```python
from build123d import *

# Parameters (mm, degrees)
SKETCH1_W                                    = 25.4
SKETCH1_H                                    = 6.35
BOSS_EXTRUDE3_DEPTH                          = 6.35
BOSS_EXTRUDE5_DEPTH                          = 6.35
CBORE_FOR_M3_HEX_SOCKET_HEAD_CAP_SCR_2_COUNT = 2
CBORE_FOR_M3_HEX_SOCKET_HEAD_CAP_SCR_2_PITCH = 50.8
CIRPATTERN1_COUNT                            = 5
F_3_0MM_DOWEL_HOLE1_D                        = 3
F_3_0MM_DOWEL_HOLE1_CSINK_D                  = 3.05
F_3_0MM_DOWEL_HOLE1_CSINK_ANGLE              = 90


with BuildPart() as part:
    # Sketch1 → Boss-Extrude3 (new body)
    with BuildSketch(Plane.XY):
        Polygon((-124.216211638, 59.788282184), (-139.456211638, 80.108282184), (-159.776211638, 64.868282184), (-144.536211638, 44.548282184), (-168.571099043, 36.333406201), (-160.356223061, 12.298518796), (-136.321335655, 20.513394779), (-128.106459673, -3.521492627), (-152.141347078, -11.73636861), (-143.926471095, -35.771256015), (-119.89158369, -27.556380032), (-111.676707707, -51.591267438), (-135.711595113, -59.80614342), (-127.49671913, -83.841030826), (-103.461831725, -75.626154843), (-95.246955742, -99.661042248), (-119.281843147, -107.875918231), (-111.066967165, -131.910805636), (-87.032079759, -123.695929654), (-86.646457092, -149.093002224), (-61.249384521, -148.707379557), (-61.635007189, -123.310306986), (-36.237934618, -122.924684318), (-35.85231195, -148.321756889), (-10.45523938, -147.936134221), (-10.840862048, -122.539061651), (14.556210523, -122.153438983), (14.941833191, -147.550511554), (40.338905761, -147.164888886), (39.953283094, -121.767816315), (65.350355664, -121.382193648), (65.735978332, -146.779266218), (91.133050903, -146.393643551), (90.747428235, -120.99657098), (115.020643556, -128.477949061), (122.502021637, -104.20473374), (98.228806316, -96.723355659), (105.710184397, -72.450140338), (129.983399717, -79.931518419), (137.464777798, -55.658303098), (113.191562477, -48.176925017), (120.672940558, -23.903709697), (144.946155879, -31.385087777), (152.42753396, -7.111872456), (128.154318639, 0.369505624), (135.63569672, 24.642720945), (159.90891204, 17.161342864), (167.390290121, 41.434558185), (143.1170748, 48.915936266), (157.733124217, 69.6892629), (136.959797583, 84.305312317), (122.343748166, 63.531985683), (101.570421532, 78.1480351), (116.186470949, 98.921361734), (95.413144315, 113.537411151), (80.797094898, 92.764084517), (60.023768264, 107.380133933), (74.639817681, 128.153460567), (53.866491047, 142.769509984), (39.25044163, 121.99618335), (18.477114996, 136.612232767), (33.093164413, 157.385559401), (12.319837779, 172.001608818), (-2.296211638, 151.228282184), (-17.536211638, 171.548282184), (-37.856211638, 156.308282184), (-22.616211638, 135.988282184), (-83.576211638, 90.268282184), (-98.816211638, 110.588282184), (-119.136211638, 95.348282184), (-103.896211638, 75.028282184), align=None)
        with Locations((-91.196211638, 3.175)):
            Rectangle(SKETCH1_W, SKETCH1_H, mode=Mode.SUBTRACT)
        with Locations((-35.316211638, 3.175)):
            Rectangle(SKETCH1_W, SKETCH1_H, mode=Mode.SUBTRACT)
        Polygon((22.412996771, 7.033712007), (47.801287728, 7.804868454), (47.99407684, 1.457795715), (22.605785883, 0.686639268), align=None, mode=Mode.SUBTRACT)
        Polygon((103.655527834, 9.501412638), (103.848316946, 3.154339898), (78.460025989, 2.383183451), (78.267236877, 8.730256191), align=None, mode=Mode.SUBTRACT)
    extrude(amount=BOSS_EXTRUDE3_DEPTH)

    # Sketch1_6 → Boss-Extrude5 (add)
    with BuildSketch(Plane.XY):
        Polygon((-78.496211638, 125.828282184), (-63.256211638, 105.508282184), (-42.936211638, 120.748282184), (-58.176211638, 141.068282184), align=None)
    extrude(amount=BOSS_EXTRUDE5_DEPTH)

    # Sketch10 → CBORE for M3 Hex Socket Head Cap Screw1 (revolve, cut)
    with BuildSketch(Plane(origin=(-60.716211638, 123.288282184, 6.35), x_dir=(0, -1, 0), z_dir=(1, 0, 0))):
        Polygon((0, 0), (0, 6.35), (1.7, 6.35), (1.7, 3.4), (3.25, 3.4), (3.25, 0.025), (3.275, 0), align=None)
    cbore_for_m3_hex_socket_head_cap_screw1 = revolve(axis=Axis((-60.716211638, 123.288282184, 12.7), (0, 0, -1)), mode=Mode.SUBTRACT)

    # CBORE for M3 Hex Socket Head Cap Scr 2: CBORE for M3 Hex Socket Head Cap Screw1 ×2
    with Locations(*[Vector(-0.8, -0.5999999999999999, 0) * (i * CBORE_FOR_M3_HEX_SOCKET_HEAD_CAP_SCR_2_PITCH) for i in range(1, CBORE_FOR_M3_HEX_SOCKET_HEAD_CAP_SCR_2_COUNT)]):
        add(cbore_for_m3_hex_socket_head_cap_screw1, mode=Mode.SUBTRACT)

    # CirPattern1: CBORE for M3 Hex Socket Head Cap Screw1 ×5 about axis
    cirpattern1_axis = Axis((0, 0, 0), (0, 0, 1))
    for i in range(1, CIRPATTERN1_COUNT):
        add(cbore_for_m3_hex_socket_head_cap_screw1.rotate(cirpattern1_axis, i * 360 / CIRPATTERN1_COUNT), mode=Mode.SUBTRACT)

    # CirPattern1 copy 1 sketch → CirPattern1 copy 1 (revolve, cut)
    with BuildSketch(Plane(origin=(-119.586713419, -67.716149132, 6.35), x_dir=(0.9510565162951535, -0.30901699437494745, 0), z_dir=(0.30901699437494745, 0.9510565162951535, 0))):
        Polygon((0, 0), (0, 6.35), (1.7, 6.35), (1.7, 3.4), (3.25, 3.4), (3.25, 0.025), (3.275, 0), align=None)
    revolve(axis=Axis((-119.586713419, -67.716149132, 12.7), (0, 0, -1)), mode=Mode.SUBTRACT)

    # CirPattern1 copy 2 sketch → CirPattern1 copy 2 (revolve, cut)
    with BuildSketch(Plane(origin=(27.447558142, -134.659163935, 6.35), x_dir=(0.5877852522924732, 0.8090169943749473, 0), z_dir=(-0.8090169943749473, 0.5877852522924732, 0))):
        Polygon((0, 0), (0, 6.35), (1.7, 6.35), (1.7, 3.4), (3.25, 3.4), (3.25, 0.025), (3.275, 0), align=None)
    revolve(axis=Axis((27.447558142, -134.659163935, 12.7), (0, 0, -1)), mode=Mode.SUBTRACT)

    # CirPattern1 copy 3 sketch → CirPattern1 copy 3 (revolve, cut)
    with BuildSketch(Plane(origin=(136.550237259, -15.507791077, 6.35), x_dir=(-0.587785252292473, 0.8090169943749476, 0), z_dir=(-0.8090169943749476, -0.587785252292473, 0))):
        Polygon((0, 0), (0, 6.35), (1.7, 6.35), (1.7, 3.4), (3.25, 3.4), (3.25, 0.025), (3.275, 0), align=None)
    revolve(axis=Axis((136.550237259, -15.507791077, 12.7), (0, 0, -1)), mode=Mode.SUBTRACT)

    # CirPattern1 copy 4 sketch → CirPattern1 copy 4 (revolve, cut)
    with BuildSketch(Plane(origin=(56.945129656, 125.074821959, 6.35), x_dir=(-0.9510565162951536, -0.30901699437494723, 0), z_dir=(0.30901699437494723, -0.9510565162951536, 0))):
        Polygon((0, 0), (0, 6.35), (1.7, 6.35), (1.7, 3.4), (3.25, 3.4), (3.25, 0.025), (3.275, 0), align=None)
    revolve(axis=Axis((56.945129656, 125.074821959, 12.7), (0, 0, -1)), mode=Mode.SUBTRACT)

    # 3.0mm Dowel Hole1 (through all)
    with Locations(Plane.XY.offset(6.35)):
        with Locations((-40.904211638, -45.212), (40.883788362, -45.212)):
            CounterSinkHole(F_3_0MM_DOWEL_HOLE1_D / 2, F_3_0MM_DOWEL_HOLE1_CSINK_D / 2, counter_sink_angle=F_3_0MM_DOWEL_HOLE1_CSINK_ANGLE)


solid = part.part
```
Model file for the job. Use its own axes, mm. A direction names the side the tool comes from. Coordinates: 2 decimals unless noted, no trailing zeros. Write item = value, one per line. Start each with the question number.
Item 1: Saw through at A-A, the plane z = 1.25. State how many separate pieces and enclosed holes the cut face has, then the cut area to 3 significant figures.
Item 2: 3-axis set-ups, long thin cutter, end or side, ignore diameter. For faces 5 (the face through (129.75, 74.06, 3.13)), 6 (the face through (-164.52, 24.48, 3.13)), 7 (the face through (-148.507, 16.348, 3.131)): which of +Z, -Z, +X, -X, +Y, -Y reach the whole face in a straight line?
Item 3: Wall check: probe 1 along X at (y, z) = (95, 3.75) (3 decimals); probe 2 along Y at (x, z) = (-36.5, 0.5); probe 3 along X at (y, z) = (63.5, 4.5). Give the ranges that are in metal, low to high. Write a range as [from, to].
Item 4: Drop flat-ended pins along their axis: pin 1 Ø1 at (x, z) = (77.5, 3.5) entering from -Y; pin 2 Ø2 at (x, y) = (121.5, -63.5) entering from +Z; pin 3 Ø3 at (x, z) = (-88.5, 4) entering from +Y; pin 4 Ø1.9 at (y, z) = (4, 4) entering from +X. Give the stop position or say it passes through.
Item 5: Pull direction X, two halves, no side cores. Call faces 1 (the face through (-111.6, 85.3, 3.1)), 2 (the face through (140.461, -3.424, 3.131)), 3 (the face through (-131.66, -71.66, 3.13)), 4 (the face through (-9.81, 161.246, 3.131)): +X half, -X half, draft (parallel to the pull), parting line (faces both ways), or undercut.
Answers:
q1.separate_pieces = 1
q1.enclosed_holes = 16
q1.area = 66,500 mm2
q2.face_5 = +Z, -Z, +Y
q2.face_6 = +Z, -Z, -X, -Y
q2.face_7 = +Z, -Z
q3.probe_1 = [-118.875, -103.756], [-98.956, -87.125], [-77.267, 77.619], [82.37, 95.353], [101.631, 113.427]
q3.probe_2 = [-122.93, 0], [6.35, 125.58], [154.5, 157.33]
q3.probe_3 = [-158.75, -127], [-119.27, 153.38]
q4.pin_1 = -146.61
q4.pin_2 = through
q4.pin_3 = 98.83
q4.pin_4 = 129.57
q5.face_1 = undercut
q5.face_2 = +X half
q5.face_3 = -X half
q5.face_4 = undercut
